Autodesk Inventor part; units mm, degrees
ref_plane "YZ Plane" through (0, 0, 0) normal (1, 0, 0) x (0, 1, 0)
ref_plane "XZ Plane" through (0, 0, 0) normal (0, 1, 0) x (-1, 0, 0)
ref_plane "XY Plane" through (0, 0, 0) normal (0, 0, 1) x (1, 0, 0)
sketch "Sketch6" plane through (0, 0, 0) normal (0, 1, 0) x (-1, 0, 0)
  line L0 (306.3, -490) -> (-306.3, -490)
  line L1 (-306.3, -490) -> (-306.3, 490)
  line L2 (-306.3, 490) -> (306.3, 490)
  line L3 (306.3, 490) -> (306.3, -490)
  line L4 (306.3, -490) -> (-306.3, 490) construction
  line L5 (-306.3, -490) -> (306.3, 490) construction
  point P0 (0, 0)
  dimension "d52" = 612.6
  dimension "d53" = 980
extrude "Plate2" add sketch "Sketch6" along normal blind 0.5
sketch "Sketch11" plane through (-305.8, 0, 490) normal (-1, 0, 0) x (0, -1, 0)
  line L0 (0, -980) -> (0, 0)
  line L1 (0, 0) -> (-10, 0)
  line L2 (-10, 0) -> (-10, -980)
  line L3 (-10, -980) -> (0, -980)
edge flange "Flange2" height 10 angle 90 thickness 0.5 bend radius 0.5 thickness toward (-1, 0, 0) relief tear relief width 0.5 relief depth 0.25 edges at (-306.3, 0.5, 0) wall of the first edge with corners at (-305.8, 0, -490) (-305.8, 0, 490) (-305.8, 10, 490) (-305.8, 10, -490)
bend "Bend3"
corner "Corner3"
sketch "Sketch12" plane through (-306.3, 9.5, 490) normal (0, 1, 0) x (-1, 0, 0)
  line L0 (0, -980) -> (0, 0)
  line L1 (0, 0) -> (-10, 0)
  line L2 (-10, 0) -> (-10, -980)
  line L3 (-10, -980) -> (0, -980)
edge flange "Flange3" height 10 angle 90 thickness 0.5 bend radius 0.5 thickness toward (0, 1, 0) relief tear relief width 0.5 relief depth 0.25 edges at (-305.8, 10, 0) wall of the first edge with corners at (-306.3, 9.5, -490) (-306.3, 9.5, 490) (-296.3, 9.5, 490) (-296.3, 9.5, -490)
bend "Bend4"
corner "Corner4"
sketch "Sketch13" plane through (305.8, 0, -490) normal (1, 0, 0) x (0, 1, 0)
  line L0 (0, 980) -> (0, 0)
  line L1 (0, 0) -> (10, 0)
  line L2 (10, 0) -> (10, 980)
  line L3 (10, 980) -> (0, 980)
edge flange "Flange4" height 10 angle 90 thickness 0.5 bend radius 0.5 thickness toward (1, 0, 0) relief tear relief width 0.5 relief depth 0.25 edges at (306.3, 0.5, 0) wall of the first edge with corners at (305.8, 0, 490) (305.8, 0, -490) (305.8, 10, -490) (305.8, 10, 490)
bend "Bend5"
corner "Corner5"
sketch "Sketch14" plane through (306.3, 9.5, -490) normal (0, 1, 0) x (-1, 0, 0)
  line L0 (0, 980) -> (0, 0)
  line L1 (0, 0) -> (10, 0)
  line L2 (10, 0) -> (10, 980)
  line L3 (10, 980) -> (0, 980)
edge flange "Flange5" height 10 angle 90 thickness 0.5 bend radius 0.5 thickness toward (0, 1, 0) relief tear relief width 0.5 relief depth 0.25 edges at (305.8, 10, 0) wall of the first edge with corners at (306.3, 9.5, 490) (306.3, 9.5, -490) (296.3, 9.5, -490) (296.3, 9.5, 490)
bend "Bend6"
corner "Corner6"
equation "\"d52\" = ЖАБРЫ_базовая_ширина - 3 * ЖАБРЫ_шаг_листов"
equation "\"d53\" = ЖАБРЫ_базовая_длина_кор_лист"
equation "\"d54\" = Thickness"
equation "\"d84\" = BendReliefWidth"
equation "\"d85\" = BendReliefDepth"
equation "\"d86\" = MinimumRemnant"
equation "\"d87\" = TransitionRadius"
equation "\"d90\" = BendRadius"
equation "\"d91\" = CornerReliefSize"
equation "\"d92\" = GapSize"
equation "\"d93\" = JacobiRadiusSize"
equation "\"d94\" = BendReliefWidth"
equation "\"d95\" = BendReliefDepth"
equation "\"d96\" = MinimumRemnant"
equation "\"d97\" = TransitionRadius"
equation "\"d100\" = BendRadius"
equation "\"d101\" = CornerReliefSize"
equation "\"d102\" = GapSize"
equation "\"d103\" = JacobiRadiusSize"
equation "\"d104\" = BendReliefWidth"
equation "\"d105\" = BendReliefDepth"
equation "\"d106\" = MinimumRemnant"
equation "\"d107\" = TransitionRadius"
equation "\"d110\" = BendRadius"
equation "\"d111\" = CornerReliefSize"
equation "\"d112\" = GapSize"
equation "\"d113\" = JacobiRadiusSize"
equation "\"d114\" = BendReliefWidth"
equation "\"d115\" = BendReliefDepth"
equation "\"d116\" = MinimumRemnant"
equation "\"d117\" = TransitionRadius"
equation "\"d120\" = BendRadius"
equation "\"d121\" = CornerReliefSize"
equation "\"d122\" = GapSize"
equation "\"d123\" = JacobiRadiusSize"
equation "\"BendRadius\" = Thickness"
equation "\"BendReliefWidth\" = Thickness"
equation "\"BendReliefDepth\" = 0.5 * Thickness"
equation "\"CornerReliefSize\" = 4 * Thickness"
equation "\"MinimumRemnant\" = 2 * Thickness"
equation "\"TransitionRadius\" = BendRadius"
equation "\"JacobiRadiusSize\" = BendRadius"
equation "\"GapSize\" = Thickness"
properties part number "MSC 807 sheet gills" material "Stainless Steel"
Input: part model. Units: mm. Frame: model coordinates. Coordinates: 2 decimals unless noted, no trailing zeros. Loops run counter-clockwise (first coordinate to the right, second up) from the corner with the lowest first, then second, coordinate; pieces in that order, holes last. Notation, with made-up numbers: (-27, -38) -> (31, -38) arc R28 ccw to (31, -14) -> close; hole circle Ø1 at (31.25, -1.5). An arc over 180 degrees is marked (long way). One line per item, written item: value.
(1) Ray query, line 1 along X through (y, z) = (8, -4); line 2 along Y through (x, z) = (242.5, 301). Return the intervals inside material, ascending.
Answer below:
line 1: x = -306.3 to -305.8, 305.8 to 306.3
line 2: y = 0 to 0.5
(2) Cut plane B-B (z = -157.5). Output: boundary loops of the cut face in (x, y).
Answer below:
outline: (-306.3, 1) arc R1 ccw to (-305.3, 0) -> (305.3, 0) arc R1 ccw to (306.3, 1) -> (306.3, 9) arc R1 ccw to (305.3, 10) -> (296.3, 10) -> (296.3, 9.5) -> (305.3, 9.5) arc R0.5 cw to (305.8, 9) -> (305.8, 1) arc R0.5 cw to (305.3, 0.5) -> (-305.3, 0.5) arc R0.5 cw to (-305.8, 1) -> (-305.8, 9) arc R0.5 cw to (-305.3, 9.5) -> (-296.3, 9.5) -> (-296.3, 10) -> (-305.3, 10) arc R1 ccw to (-306.3, 9) -> close
(3) Cut plane A-A (y = 6.75). Output: boundary loops of the cut face in (x, z), then the cut area to 3 significant figures.
Answer below:
outline: (-306.3, -490) -> (-305.8, -490) -> (-305.8, 490) -> (-306.3, 490) -> close; (305.8, -490) -> (306.3, -490) -> (306.3, 490) -> (305.8, 490) -> close
area: 980 mm2
(4) Draft query along X for faces 1 (the face through (4, 0.5, 7)), 2 (the face through (4, 0, 7)). Return one class per face: pulls with the +X half, pulls with the -X half, needs draft (parallel to the pull), parting line crosses it, or undercut.
Answer below:
face 1: undercut
face 2: needs draft
(5) Pin query (flat end, axial travel): pin 1 Ø6 at (x, z) = (176, 252.5) entering from +Y; pin 2 Ø0.6 at (y, z) = (10, -73.5) entering from +X. Return the tip coordinate at first contact, or that it passes through.
Answer below:
pin 1: stops at y = 0.5
pin 2: stops at x = 306.01
(6) Cut plane C-C (x = 114). Output: boundary loops of the cut face in (y, z).
Answer below:
outline: (0, -490) -> (0.5, -490) -> (0.5, 490) -> (0, 490) -> close
